from build123d import *

# Parameters (mm, degrees)
SKETCH1_W               = 150
SKETCH1_H               = 60
BOSS_EXTRUDE1_DEPTH     = 3
SKETCH2_W               = 3
SKETCH2_H               = 10
CUT_EXTRUDE1_DEPTH      = 81.833161512
LPATTERN1_COUNT         = 3
LPATTERN1_PITCH         = 20
MIRROR1_COPY_1_SKETCH_W = 3
MIRROR1_COPY_1_SKETCH_H = 10
MIRROR1_COPY_1_DEPTH    = 81.833161512
MIRROR1_COPY_2_SKETCH_W = 3
MIRROR1_COPY_2_SKETCH_H = 10
MIRROR1_COPY_2_DEPTH    = 81.833161512
SKETCH3_W               = 10
SKETCH3_H               = 3
CUT_EXTRUDE2_DEPTH      = 81.833161512
LPATTERN2_COUNT         = 7
LPATTERN2_PITCH         = 20


with BuildPart() as part:
    # Sketch1 → Boss-Extrude1 (new body)
    with BuildSketch(Plane(origin=(0, 0, 0), x_dir=(1, 0, 0), z_dir=(0, 1, 0))):
        Rectangle(SKETCH1_W, SKETCH1_H)
    extrude(amount=BOSS_EXTRUDE1_DEPTH)

    # Sketch2 → Cut-Extrude1 (cut, through all)
    with BuildSketch(Plane(origin=(0, 3, 0), x_dir=(1, 0, 0), z_dir=(0, 1, 0))):
        with Locations((73.5, -15)):
            Rectangle(SKETCH2_W, SKETCH2_H)
    cut_extrude1 = extrude(amount=-CUT_EXTRUDE1_DEPTH, mode=Mode.SUBTRACT)

    # LPattern1: Cut-Extrude1 ×3
    with Locations(*[(0, 0, -i * LPATTERN1_PITCH) for i in range(1, LPATTERN1_COUNT)]):
        add(cut_extrude1, mode=Mode.SUBTRACT)

    # Mirror1: Cut-Extrude1 across plane
    add(cut_extrude1.mirror(Plane(origin=(0, 0, 0), x_dir=(0, 0, 1), z_dir=(1, 0, 0))), mode=Mode.SUBTRACT)

    # Mirror1 copy 1 sketch → Mirror1 copy 1 (cut, through all)
    with BuildSketch(Plane(origin=(0, 3, -20), x_dir=(-1, 0, 0), z_dir=(0, 1, 0))):
        with Locations((73.5, 15)):
            Rectangle(MIRROR1_COPY_1_SKETCH_W, MIRROR1_COPY_1_SKETCH_H)
    extrude(amount=-MIRROR1_COPY_1_DEPTH, mode=Mode.SUBTRACT)

    # Mirror1 copy 2 sketch → Mirror1 copy 2 (cut, through all)
    with BuildSketch(Plane(origin=(0, 3, -40), x_dir=(-1, 0, 0), z_dir=(0, 1, 0))):
        with Locations((73.5, 15)):
            Rectangle(MIRROR1_COPY_2_SKETCH_W, MIRROR1_COPY_2_SKETCH_H)
    extrude(amount=-MIRROR1_COPY_2_DEPTH, mode=Mode.SUBTRACT)

    # Sketch3 → Cut-Extrude2 (cut, through all)
    with BuildSketch(Plane(origin=(0, 3, 0), x_dir=(1, 0, 0), z_dir=(0, 1, 0))):
        with Locations((-60, 28.5)):
            Rectangle(SKETCH3_W, SKETCH3_H)
    cut_extrude2 = extrude(amount=-CUT_EXTRUDE2_DEPTH, mode=Mode.SUBTRACT)

    # LPattern2: Cut-Extrude2 ×7
    with Locations(*[(i * LPATTERN2_PITCH, 0, 0) for i in range(1, LPATTERN2_COUNT)]):
        add(cut_extrude2, mode=Mode.SUBTRACT)


solid = part.part
Input: part model. Units: mm. Frame: model coordinates. A direction names the side the tool comes from. Coordinates: 2 decimals unless noted, no trailing zeros. Loops run counter-clockwise (first coordinate to the right, second up) from the corner with the lowest first, then second, coordinate; pieces in that order, holes last. Notation, with made-up numbers: (47, -24) -> (76, -24) arc R22 ccw to (76, 11) -> close; hole circle Ø5 at (77.25, 38). An arc over 180 degrees is marked (long way). Write each question's results on one line, items separated by ' | '. Start each with the question number.
Q1. Reachability of faces 4 (the flat face through (-25, 2, -28)), 5 (the flat face through (-75, 1, 5)), 6 (the flat face through (-72, 2, -25)), 7 (the flat face through (73, 2, -10)), 8 (the flat face through (73, 2, -20)) from +Z, -Z, +X, -X, +Y, -Y: full face, straight path, thin tool, end or side. Return the list, or none.
Q2. Pull-direction query (Z, two-part tool) for faces 1 (the flat face through (-10, 1, -30)), 2 (the flat face through (73, 2, 0)), 3 (the flat face through (45, 2, -28)); classes: released by +Z, released by -Z, zero draft, split by the parting line, or undercut.
Q3. Section B-B, the plane x = 2. Return the cut outline in (y, z), plus the area to 3 significant figures.
Q4. Section A-A, the plane z = -7. Return the cut outline in (x, y), plus the area to 3 significant figures.
Q5. Ray query, line 1 (X direction, y = 2.85, z = -26.5); line 2 (Z direction, x = 15.5, y = 0.7). Return the intervals inside material, ascending. Write a range as from..to.
Q6. Pin query (flat end, axial travel): pin 1 (0.9 mm diameter, centred on y = 1, z = -28.5, fed in from -X); pin 2 (0.9 mm diameter, centred on x = 0.5, y = 1.5, fed in from -Z); pin 3 (1.5 mm diameter, centred on y = 2, z = -28, fed in from +X). Return the tip coordinate at first contact, or that it passes through.
Found:
1) face 4: -Z, +Y, -Y | face 5: +Z, -Z, -X, +Y, -Y | face 6: -Z, -X, +Y, -Y | face 7: +X, +Y, -Y | face 8: -Z, +X, +Y, -Y
2) face 1: released by -Z | face 2: undercut | face 3: zero draft
3) outline: (0, -27) -> (3, -27) -> (3, 30) -> (0, 30) -> close | area: 171 mm2
4) outline: (-72, 0) -> (72, 0) -> (72, 3) -> (-72, 3) -> close | area: 432 mm2
5) line 1: -72..72 | line 2: -27..30
6) pin 1: x = -72 | pin 2: z = -27 | pin 3: x = 72
